from build123d import *

# Parameters (mm, degrees)
F0_R     = 7
F0_R_2   = 5.2
F1_DEPTH = 9
F0_R_3   = 8
F2_DEPTH = 1
F3_R     = 8
F3_R_2   = 7
F4_DEPTH = 1
F5_SIZE  = 0.99999


# Not quite as in the source:
# - a fillet or chamfer is up to 0.001 mm smaller than in the source, because OpenCascade refuses the exact size


with BuildPart() as f1:
    # F0 (on Top) → F1 (new body)
    with BuildSketch(Plane.XY):
        Circle(F0_R)
        Circle(F0_R_2, mode=Mode.SUBTRACT)
    extrude(amount=F1_DEPTH)

    # F0 (on Top) → F2 (join)
    with BuildSketch(Plane.XY):
        Circle(F0_R_3)
        Circle(F0_R, mode=Mode.SUBTRACT)
    extrude(amount=F2_DEPTH)

    # F3 (on face) → F4 (join)
    with BuildSketch(Plane.XY.offset(9)):
        Circle(F3_R)
        Circle(F3_R_2, mode=Mode.SUBTRACT)
    extrude(amount=-F4_DEPTH)

    # F5 (size 1 in the source; OpenCascade refuses exactly that, so slightly less here)
    f5_edges = [f1.edges().sort_by_distance(p)[0] for p in [
        (-8, 0, 8),
        (-8, 0, 1),
    ]]
    chamfer(f5_edges, length=F5_SIZE)


solid = f1.part
The model under review builds one solid part; all positions refer to its coordinate system, in mm. Give positions to 0.01 mm unless a question says otherwise; leave off trailing zeros. Order: outer loops, then holes, each group sorted by start corner. A loop starts at its lowest first (then second) coordinate and runs counter-clockwise, first axis right, second up. Notation, with made-up numbers: M 10,12 L 53,12 A36 ccw 53,50 Z; hole C 34.5,26.5 d6. An arc over 180 degrees is marked long. Use one line per item in the form item = value. Start each with the question number.
Item 1: We need section C-C on z = 7.25. Give the boundary of the cut face in (x, y), plus the area to 3 significant figures.
Item 2: The part is to be moulded in two halves that separate along Z. For faces 1 (the flat face through (5, -2, 9)), 2 (the cylindrical face through (-0.677, 5.156, 4.437)), 3 (the cylindrical face through (6.466, -2.681, 4.451)), say which applies: pulls with the +Z half, pulls with the -Z half, needs draft (parallel to the pull), parting line crosses it, or undercut.
Item 3: To check wall thickness, follow line 1 along Y through (x, z) = (3.75, 2.5); line 2 along Z through (x, y) = (-3.25, -6.25); line 3 along X through (y, z) = (1.5, 1.5). State the ranges of each line that lie inside material, in increasing order. Write a range as from..to.
Item 4: Insertion check: pin 1 Ø4 at (x, y) = (0, 2.5) entering from -Z; pin 2 Ø4 at (x, z) = (2.5, 4) entering from -Y; pin 3 Ø3 at (x, z) = (-0.5, 2) entering from -Y; pin 4 Ø1 at (x, z) = (-1.5, 3.5) entering from +Y. Each pin has a flat end and moves straight along its axis. Give the tip position at first contact, or say it passes through.
Completed:
q1.outline = C 0,0 d14; hole C 0,0 d10.4
q1.area = 69.0 mm²
q2.face_1 = pulls with the +Z half
q2.face_2 = needs draft
q2.face_3 = undercut
q3.line_1 = -5.91..-3.6, 3.6..5.91
q3.line_2 = 0..0.96, 8.04..9
q3.line_3 = -6.84..-4.98, 4.98..6.84
q4.pin_1 = through
q4.pin_2 = -6.98
q4.pin_3 = -7.49
q4.pin_4 = 6.93
